from build123d import *

# Parameters (mm, degrees)
CUT_EXTRUDE1_DEPTH      = 395.646626743
CUT_EXTRUDE1_DEPTH_BACK = 395.646626743
SKETCH2_W               = 193.8
SKETCH2_H               = 31.1
CUT_EXTRUDE2_DEPTH      = 396.001126581
CUT_EXTRUDE2_DEPTH_BACK = 396.001126581
SKETCH3_R               = 6.25


with BuildPart() as part:
    # Sketch1 → Revolve1 (revolve)
    with BuildSketch(Plane.XY, mode=Mode.PRIVATE) as revolve1_sk:
        Polygon((0, 0), (0, 28), (-247.1, 28), (-247.1, 43.6), (-271.1, 43.6), (-271.1, 18.75), (-360.9, 18.75), (-360.9, 7.796453039), (-386.8, 7.796453039), (-389.8, 4.796453039), (-389.8, 0), align=None)
    revolve(revolve1_sk.sketch.rotate(Axis((0, 0, 0), (-1, 0, 0)), 90), axis=Axis((0, 0, 0), (-1, 0, 0)))

    # Sketch2 → Cut-Extrude1 (cut, two sides: drawn at the far end of the back side and taken through both)
    with BuildSketch(Plane.XY.offset(-CUT_EXTRUDE1_DEPTH_BACK)):
        with Locations((-112, 12.45)):
            Rectangle(SKETCH2_W, SKETCH2_H)
    extrude(amount=CUT_EXTRUDE1_DEPTH + CUT_EXTRUDE1_DEPTH_BACK, mode=Mode.SUBTRACT)

    # Sketch3 → Cut-Extrude2 (cut, two sides: drawn at the far end of the back side and taken through both)
    with BuildSketch(Plane(origin=(0, -3.1, 0), x_dir=(1, 0, 0), z_dir=(0, 1, 0)).offset(-CUT_EXTRUDE2_DEPTH_BACK)):
        with Locations(Location((-162, -0.172136266, 0), (0, 0, 180))):
            Circle(SKETCH3_R)
        with Locations(Location((-62, -0.172136266, 0), (0, 0, 180))):
            Circle(SKETCH3_R)
    extrude(amount=CUT_EXTRUDE2_DEPTH + CUT_EXTRUDE2_DEPTH_BACK, mode=Mode.SUBTRACT)


solid = part.part
Here's how the part is built. I have some questions about the finished solid (model axes, mm). A direction names the side the tool comes from. Coordinates: 2 decimals unless noted, no trailing zeros. Write each loop counter-clockwise with the first axis right and the second up, starting at its lowest first coordinate (ties: lowest second). Pieces come first, ordered by that corner, then holes. Notation, with made-up numbers: (82.25, -21.75) - (100.25, -21.75) arc R18 ccw to (100.25, 7.25) - close; hole circle Ø11 at (-20.5, 4.25). An arc over 180 degrees is marked (long way). Use one line per item in the form item = value.
1) Suppose I cut it at C-C, the plane y = -33. Write out the boundary of the cut face in (x, z).
Solved:
outline = (-271.1, -28.49) - (-247.1, -28.49) - (-247.1, 28.49) - (-271.1, 28.49) - close
2) Thinking about a two-plate mould opening in Z: for faces 5 (the flat face through (-208.9, 9, 0)), 6 (the cylindrical face through (-167.96, -15.73, 2.05)), 7 (the cylindrical face through (-259.27, 38.68, -20.12)), which applies, released by +Z, released by -Z, zero draft, split by the parting line, or undercut?
Solved:
face_5 = zero draft
face_6 = undercut
face_7 = split by the parting line
3) Suppose I cut it at B-B, the plane x = -162. Write out the boundary of the cut face in (y, z).
Solved:
outline = (-27.33, -6.08) arc R28 ccw to (-3.1, -27.83) - (-3.1, -6.08) - close; (-27.25, 6.42) - (-3.1, 6.42) - (-3.1, 27.83) arc R28 ccw to start
4) I'm going to push flat-ended pins straight in: P1, Ø8, axis at x = -231.5, y = 27.5, coming from the +Z side; P2, Ø4, axis at x = -256.5, y = 31, coming from the +Z side; P3, Ø6, axis at y = -6, z = -22, coming from the -X side; P4, Ø11, axis at x = -162, z = 0.17, coming from the +Y side. Where does each tip first touch, or does it pass through?
Solved:
P1 = 15.22
P2 = 32.56
P3 = -271.1
P4 = through
5) I need wall thicknesses on line 1 (X direction, y = 24.5, z = 1); line 2 (X direction, y = -26.5, z = -1.5); line 3 (X direction, y = 12, z = 13). Which ranges of each line are inside material? Lowest first, please.
Solved:
line_1 = -271.1 to -208.9, -15.1 to 0
line_2 = -271.1 to -168.02, -155.98 to -68.02, -55.98 to 0
line_3 = -360.9 to -208.9, -15.1 to 0
6) On a 3-axis mill with a long thin cutter (end or side, diameter ignored), from which of +Z, -Z, +X, -X, +Y, -Y can I reach the whole of each face in a straight line? I mean faces 1 (the flat face through (-247.1, 28.5, -0.6)), 2 (the cylindrical face through (-374.031, -6.574, -4.191)), 3 (the flat face through (-113, -3.1, 0)), 4 (the cylindrical face through (-67.96, -15.73, 2.05)). Say none if no direction works.
Solved:
face_1 = +X
face_2 = -X
face_3 = +Z, -Z, +Y
face_4 = +Y, -Y
7) Suppose I cut it at A-A, the plane x = -285. Write out the boundary of the cut face in (y, z), plus the area to 3 significant figures.
Solved:
outline = circle Ø37.5 at (0, 0)
area = 1,100 mm2
8) Suppose I cut it at D-D, the plane x = -41. Write out the boundary of the cut face in (y, z), plus the area to 3 significant figures.
Solved:
outline = (-3.1, -27.83) - (-3.1, 27.83) arc R28 ccw to start
area = 1,060 mm2
